The listing builds one solid part. Answer for the finished solid, in the listing's coordinates (mm). Face numbers are marked on the shaded views. A direction names the side the tool comes from. Coordinates: 2 decimals unless noted, no trailing zeros. Write each loop counter-clockwise with the first axis right and the second up, starting at its lowest first coordinate (ties: lowest second). Pieces come first, ordered by that corner, then holes.
(1) Which of the six approach directions +Z, -Z, +X, -X, +Y, -Y give full straight-line access (tool end or side, diameter ignored) to the marked faces 1, 2, 3 and 4?
(2) The part is cut by section C-C on y = 10.75. Determine the outline of the cut face in (x, z), plus the area to 3 significant figures.
(3) Given P1, Ø0.9, axis at x = 4, y = -4, coming from the -Z side; P2, Ø0.8, axis at y = -4.5, z = 4, coming from the -X side; P3, Ø1.5, axis at x = 5, z = 1, coming from the -Y side; P4, Ø2.5, axis at x = 4, y = -1.5, coming from the +Z side, each flat-ended and moving along its own axis, determine where each tip first touches the part or whether it passes through.
(4) The part is cut by section D-D on z = -0.25. Determine the outline of the cut face in (x, y).
(5) The part is cut by section B-B on x = 1. Determine the outline of the cut face in (y, z), plus the area to 3 significant figures.
(6) Straight lines are drawn through the part: line 1 (Z direction, x = 3.75, y = 10.5); line 2 (Z direction, x = 0.5, y = -0.25); line 3 (Z direction, x = 1.5, y = -4.5) (3 decimals). For each, find the intervals that lie inside material, in ascending order.
(7) The part is cut by section A-A on z = 3.75. Determine the outline of the cut face in (x, y), plus the area to 3 significant figures.
from build123d import *

# Parameters (mm, degrees)
SKETCH1_W                = 5.9944
SKETCH1_H                = 12.8016
BOSS_EXTRUDE1_DEPTH      = 0.127
BOSS_EXTRUDE2_DEPTH      = 0.8509
BOSS_EXTRUDE2_DEPTH_BACK = 0.8509
SKETCH2_W                = 7.0104
SKETCH2_H                = 5.0038
BOSS_EXTRUDE3_DEPTH      = 1.27
BOSS_EXTRUDE3_DEPTH_BACK = 1.27
SKETCH3_R                = 2.75
BOSS_EXTRUDE4_DEPTH      = 7.0104
SKETCH5_W                = 1.800661627
SKETCH5_H                = 4.2799
SKETCH5_W_2              = 1.783476746
CUT_EXTRUDE1_DEPTH       = 7.0104


with BuildPart() as part:
    # Sketch1 → Boss-Extrude1 (new body)
    with BuildSketch(Plane.XY):
        with Locations((2.9972, 6.4008)):
            Rectangle(SKETCH1_W, SKETCH1_H)
    extrude(amount=BOSS_EXTRUDE1_DEPTH)

    # Sketch2 → Boss-Extrude2 (add, two sides: drawn at the far end of the back side and taken through both)
    with BuildSketch(Plane.XY.offset(0.127).offset(-BOSS_EXTRUDE2_DEPTH_BACK)):
        with Locations((2.9972, -2.5019)):
            Rectangle(SKETCH2_W, SKETCH2_H)
    extrude(amount=BOSS_EXTRUDE2_DEPTH + BOSS_EXTRUDE2_DEPTH_BACK)

    # Sketch3 → Boss-Extrude3 (add, two sides: drawn at the far end of the back side and taken through both)
    with BuildSketch(Plane.XY.offset(0.127).offset(-BOSS_EXTRUDE3_DEPTH_BACK)):
        with Locations((2.9972, 10.0516)):
            Circle(SKETCH3_R)
    extrude(amount=BOSS_EXTRUDE3_DEPTH + BOSS_EXTRUDE3_DEPTH_BACK)

    # Sketch4 → Boss-Extrude4 (add)
    with BuildSketch(Plane.ZY.offset(0.508)):
        Polygon((0.9779, -3.3147), (4.445, -3.3147), (4.445, -5.123816362), (5.2578, -5.123816362), (5.2578, -2.5019), (0.9779, -2.5019), align=None)
    extrude(amount=-BOSS_EXTRUDE4_DEPTH)

    # Sketch5 → Cut-Extrude1 (cut)
    with BuildSketch(Plane(origin=(0, -2.5019, 0), x_dir=(1, 0, 0), z_dir=(0, 1, 0))):
        with Locations((0.392330813, -3.11785)):
            Rectangle(SKETCH5_W, SKETCH5_H)
        with Locations((2.9972, -3.11785)):
            Rectangle(SKETCH5_W_2, SKETCH5_H)
        with Locations((5.602069187, -3.11785)):
            Rectangle(SKETCH5_W, SKETCH5_H)
    extrude(amount=-CUT_EXTRUDE1_DEPTH, mode=Mode.SUBTRACT)


solid = part.part
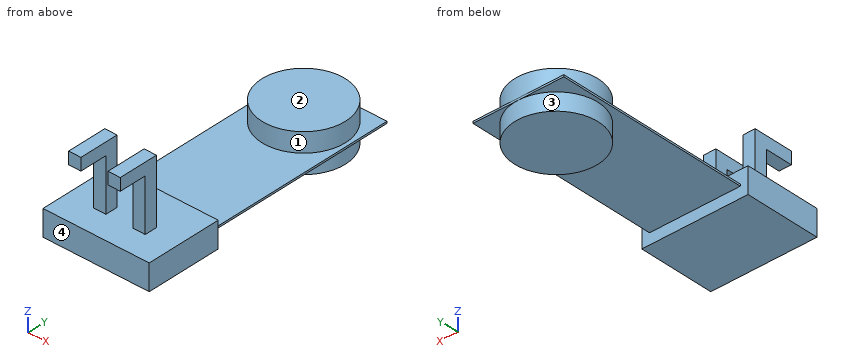
Model answer:
1. face 1: +Z
1. face 2: +Z, +X, -X, +Y
1. face 3: -Z
1. face 4: -Z, +X, -X, -Y
2. outline: (0, 0) - (0.34, 0) - (0.34, -1.14) - (5.66, -1.14) - (5.66, 0) - (5.99, 0) - (5.99, 0.13) - (5.66, 0.13) - (5.66, 1.4) - (0.34, 1.4) - (0.34, 0.13) - (0, 0.13) - close
2. area: 13.6 mm2
3. P1: stops at z = -0.72
3. P2: passes through
3. P3: stops at y = -5
3. P4: stops at z = 5.26
4. outline: (-0.51, -5) - (6.5, -5) - (6.5, 0) - (-0.51, 0) - close; circle Ø5.5 at (3, 10.05)
5. outline: (-5, -0.72) - (0, -0.72) - (0, 0) - (8.16, 0) - (8.16, -1.14) - (11.94, -1.14) - (11.94, 0) - (12.8, 0) - (12.8, 0.13) - (11.94, 0.13) - (11.94, 1.4) - (8.16, 1.4) - (8.16, 0.13) - (0, 0.13) - (0, 0.98) - (-5, 0.98) - close
5. area: 19.3 mm2
6. line 1: z = -1.14 to 1.4
6. line 2: z = -0.72 to 0.98
6. line 3: z = -0.724 to 0.978, 4.445 to 5.258
7. outline: (1.29, -3.31) - (2.11, -3.31) - (2.11, -2.5) - (1.29, -2.5) - close; (3.89, -3.31) - (4.7, -3.31) - (4.7, -2.5) - (3.89, -2.5) - close
7. area: 1.32 mm2
